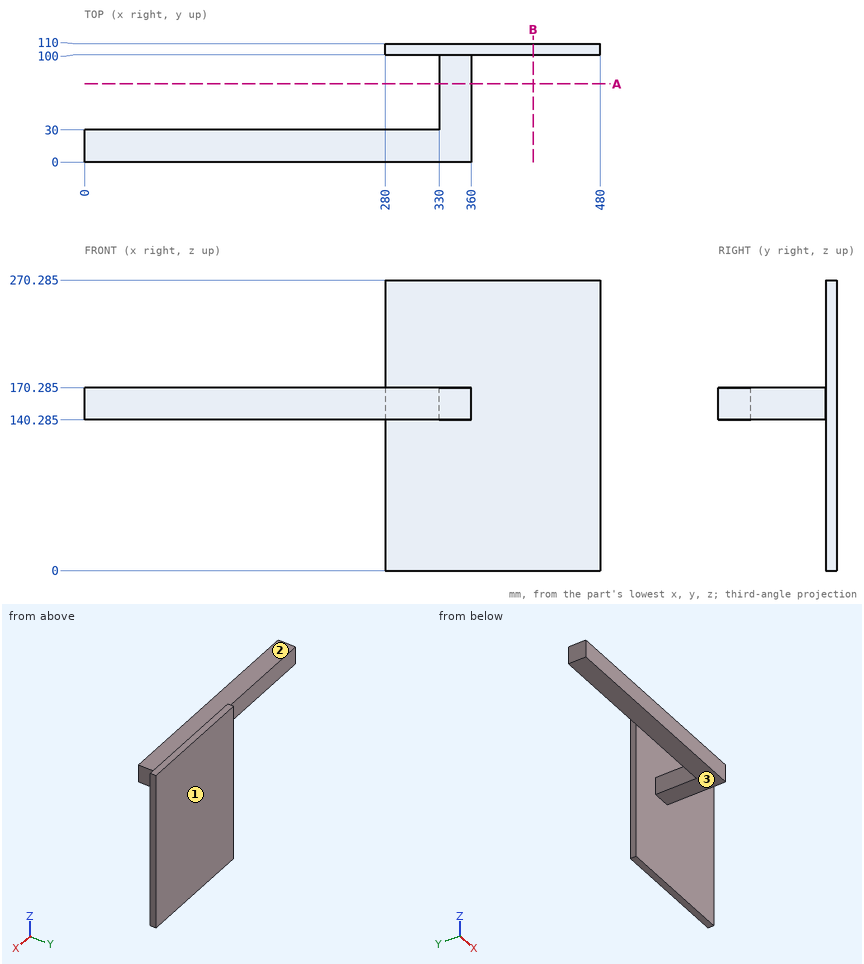
Can you work these out from the drawing? Everything is in mm from the part's minimum corner. A direction names the side the tool comes from. Round coordinates to 2 decimals unless told otherwise and drop trailing zeros. Loops run counter-clockwise (first coordinate to the right, second up) from the corner with the lowest first, then second, coordinate; pieces in that order, holes last. Notation, with made-up numbers: (83.5, -31.75) - (99.5, -31.75) arc R14 ccw to (99.5, -4.75) - close; hole circle Ø3 at (28.25, 65.25). An arc over 180 degrees is marked (long way). Answer in a Markdown table with one row per item. Add a question column.
(1) I need wall thicknesses on line 1 along Z through (x, y) = (212, 11) (1 decimal); line 2 along Y through (x, z) = (363, 179); line 3 along Y through (x, z) = (177, 141). Which ranges of each line are inside material? Lowest first, please.
(2) For the marked faces 1, 2 and 3, which set-ups out of +Z, -Z, +X, -X, +Y, -Y let a thin tool reach every point of the face, with its end or its side?
(3) If we section it at B-B (x = 417.5): Please give me the cut outline in (y, z) (1 decimal), plus the area to 3 significant figures.
(4) If we section it at A-A (y = 73): Please give me the cut outline in (x, z) (1 decimal), plus the area to 3 significant figures.
(5) I'm going to push flat-ended pins straight in: pin 1 (24 mm diameter, centred on y = 40, z = 149, fed in from +X); pin 2 (5 mm diameter, centred on y = 107.5, z = 187.5, fed in from -X); pin 3 (8 mm diameter, centred on x = 324, y = 13.5, fed in from +Z) (3 decimals). Where does each tip first touch, or does it pass through?
Model answer:
| question | item | result |
|---|---|---|
| 1 | line 1 | z = 140.3 to 170.3 |
| 1 | line 2 | y = 100 to 110 |
| 1 | line 3 | y = 0 to 30 |
| 2 | face 1 | +Z, -Z, +X, -X, +Y |
| 2 | face 2 | +Z, +X, -X, -Y |
| 2 | face 3 | -Z, +X, -X, -Y |
| 3 | outline | (100, 0) - (110, 0) - (110, 270.3) - (100, 270.3) - close |
| 3 | area | 2,700 mm² |
| 4 | outline | (330, 140.3) - (360, 140.3) - (360, 170.3) - (330, 170.3) - close |
| 4 | area | 900 mm² |
| 5 | pin 1 | stops at x = 360 |
| 5 | pin 2 | stops at x = 280 |
| 5 | pin 3 | stops at z = 170.285 |
